Autodesk Inventor part; units mm, degrees
ref_plane "YZ Plane" through (0, 0, 0) normal (1, 0, 0) x (0, 1, 0)
ref_plane "XZ Plane" through (0, 0, 0) normal (0, 1, 0) x (-1, 0, 0)
ref_plane "XY Plane" through (0, 0, 0) normal (0, 0, 1) x (1, 0, 0)
sketch "Sketch1" plane through (0, 0, 0) normal (0, 0, 1) x (1, 0, 0)
  circle A0 centre (0, 0) radius 25
  dimension "d6" = 50
extrude "Extrusion1" add sketch "Sketch1" along normal mid plane 17.58
fillet "Fillet1" radius 3 2 edges at (-25, 0, 8.79) (-25, 0, -8.79)
sketch "Sketch2" plane through (0, 0, 8.79) normal (0, 0, 1) x (1, 0, 0)
  circle A0 centre (0, 0) radius 1.5
  dimension "d10" = 3
extrude "Extrusion2" cut sketch "Sketch2" along normal through all both and the other way through all
properties part number "B-50mWheel"
Verification items for the finished model (mm, model axes). Round coordinates to 2 decimals unless told otherwise and drop trailing zeros. Write each loop counter-clockwise with the first axis right and the second up, starting at its lowest first coordinate (ties: lowest second). Pieces come first, ordered by that corner, then holes. Notation, with made-up numbers: (28, 15.25) -> (69, 15.25) arc R12 cw to (69, 28.25) -> close; hole circle Ø2 at (17.5, -16.75). An arc over 180 degrees is marked (long way). Write each question's results on one line, items separated by ' | '.
Q1. Sectioned sample at C-C, the plane z = 3.25. Record the boundary of the cut face in (x, y), and give its area (3 significant figures).
Derived:
outline: circle Ø50 at (0, 0); hole circle Ø3 at (0, 0) | area: 1,960 mm²
Q2. Sectioned sample at D-D, the plane z = -6.75. Record the boundary of the cut face in (x, y), and give its area (3 significant figures).
Derived:
outline: circle Ø49.68 at (0, 0); hole circle Ø3 at (0, 0) | area: 1,930 mm²
Q3. Draft check along X on faces 1 (the face through (23.846, 7.509, 0.081)), 2 (the face through (-1.5, 0.07, 0.12)), 3 (the face through (0, -5, -8.79)). Enter one of: released by +X, released by -X, zero draft, split by the parting line, or undercut.
Derived:
face 1: split by the parting line | face 2: undercut | face 3: zero draft
Q4. Go/stop test with flat-tipped pins: pin 1 Ø8 at (y, z) = (-16.5, 0.5) entering from +X; pin 2 Ø8 at (x, z) = (6, 5.5) entering from +Y; pin 3 Ø3 at (x, z) = (19, 4) entering from +Y. Record where each tip stops, or that it passes through.
Derived:
pin 1: stops at x = 21.65 | pin 2: stops at y = 24.92 | pin 3: stops at y = 17.85
Q5. Sectioned sample at A-A, the plane x = 0. Record the boundary of the cut face in (y, z), and give its area (3 significant figures).
Derived:
outline: (-25, -5.79) arc R3 ccw to (-22, -8.79) -> (-1.5, -8.79) -> (-1.5, 8.79) -> (-22, 8.79) arc R3 ccw to (-25, 5.79) -> close; (1.5, -8.79) -> (22, -8.79) arc R3 ccw to (25, -5.79) -> (25, 5.79) arc R3 ccw to (22, 8.79) -> (1.5, 8.79) -> close | area: 819 mm²
Q6. Thickness scan on probe 1 along Y at (x, z) = (0, 5.25); probe 2 along Y at (x, z) = (-16, 3.5); probe 3 along Z at (x, y) = (-20.5, -10.5). Record the ranges inside material, lowest first.
Derived:
probe 1: y = -25 to -1.5, 1.5 to 25 | probe 2: y = -19.21 to 19.21 | probe 3: z = -8.61 to 8.61
